The model under review builds one solid part; all positions refer to its coordinate system, in mm. Round coordinates to 2 decimals unless told otherwise and drop trailing zeros. Order: outer loops, then holes, each group sorted by start corner. A loop starts at its lowest first (then second) coordinate and runs counter-clockwise, first axis right, second up.
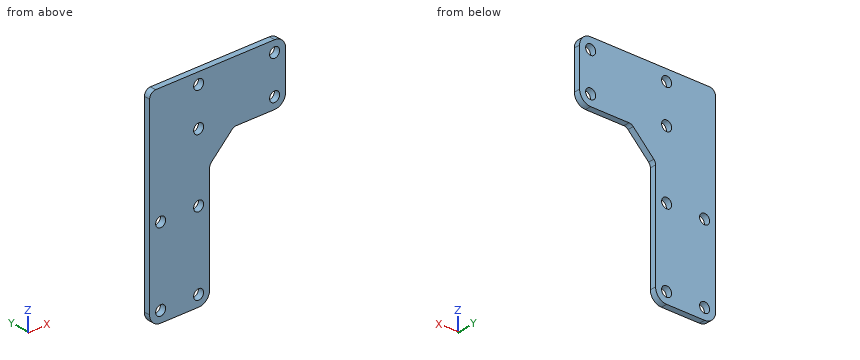
Autodesk Inventor part; units mm, degrees
ref_plane "YZ Plane" through (0, 0, 0) normal (1, 0, 0) x (0, 1, 0)
ref_plane "XZ Plane" through (0, 0, 0) normal (0, 1, 0) x (-1, 0, 0)
ref_plane "XY Plane" through (0, 0, 0) normal (0, 0, 1) x (1, 0, 0)
sketch "Sketch1" plane through (0, 0, 0) normal (0, 1, 0) x (-1, 0, 0)
  circle A0 centre (0, 0) radius 2.63
  line L0 (0, 0) -> (0, -2.63) construction
  line L1 (0, 0) -> (-2.63, 0) construction
  circle A1 centre (0, -20) radius 2.63
  circle A2 centre (-20, 0) radius 2.63 construction
  circle A3 centre (-20, -20) radius 2.63 construction
  circle A4 centre (-40, 0) radius 2.63
  circle A5 centre (-40, -20) radius 2.63
  circle A6 centre (0, -55) radius 2.63
  circle A7 centre (20, -55) radius 2.63
  circle A8 centre (20, -95) radius 2.63
  circle A9 centre (0, -95) radius 2.63
  circle A10 centre (0, 0) radius 5.805 construction
  circle A11 centre (20, -55) radius 5.805 construction
  circle A12 centre (0, -55) radius 5.805 construction
  circle A13 centre (20, -95) radius 5.805 construction
  circle A14 centre (0, -95) radius 5.805 construction
  circle A15 centre (-40, -20) radius 5.805 construction
  circle A16 centre (-40, 0) radius 5.805 construction
  line L2 (25.805, -95) -> (25.805, 2.63)
  line L3 (22.63, 5.805) -> (-40, 5.805)
  line L4 (-45.805, 0) -> (-45.805, -20)
  line L5 (-19.8201, -25.805) -> (-40, -25.805)
  circle A17 centre (-20, -20) radius 5.805 construction
  line L6 (-5.805, -39.8201) -> (-5.805, -95)
  line L7 (20, -100.805) -> (0, -100.805)
  arc A18 (20, -100.805) -> (25.805, -95) centre (20, -95) ccw
  arc A19 (-5.805, -95) -> (0, -100.805) centre (0, -95) ccw
  arc A20 (-45.805, -20) -> (-40, -25.805) centre (-40, -20) ccw
  arc A21 (-40, 5.805) -> (-45.805, 0) centre (-40, 0) ccw
  line L8 (-6.7349, -37.5751) -> (-17.5751, -26.7349)
  arc A22 (-5.805, -39.8201) -> (-6.7349, -37.5751) centre (-8.98, -39.8201) ccw
  arc A23 (-17.5751, -26.7349) -> (-19.8201, -25.805) centre (-19.8201, -28.98) ccw
  arc A24 (25.805, 2.63) -> (22.63, 5.805) centre (22.63, 2.63) ccw
  point P0 (0, -22.63)
  point P1 (-2.63, -20)
  point P2 (-20, -2.63)
  point P3 (-22.63, 0)
  point P4 (-20, -22.63)
  point P5 (-22.63, -20)
  point P6 (-40, -2.63)
  point P7 (-42.63, 0)
  point P8 (-40, -22.63)
  point P9 (-42.63, -20)
  point P10 (-5.805, -25.805)
  point P11 (-5.805, -38.505)
  point P12 (-18.505, -25.805)
  dimension "d0" = 5.26
  dimension "d3" = 20
  dimension "d6" = 20
  dimension "d10" = 20
  dimension "d12" = 75
  dimension "d13" = 40
  dimension "d14" = 3.175
  dimension "d16" = 12.7
  dimension "d17" = 12.7
  dimension "d18" = 3.175
extrude "Extrusion1" add sketch "Sketch1" along normal blind 3.175
properties part number "CNC-013-ZAxisMainMount" material "Aluminum 6061"
(1) To check wall thickness, follow probe 1 along Z at (x, y) = (0, 2.4) (3 decimals); probe 2 along Z at (x, y) = (-20, 0.95) (3 decimals); probe 3 along Z at (x, y) = (40, 2.5) (3 decimals). State the ranges of each line that lie inside material, in increasing order.
Data:
probe 1: z = -100.805 to -97.63, -92.37 to -57.63, -52.37 to -22.63, -17.37 to -2.63, 2.63 to 5.805
probe 2: z = -100.805 to -97.63, -92.37 to -57.63, -52.37 to 5.805
probe 3: z = -25.805 to -22.63, -17.37 to -2.63, 2.63 to 5.805
(2) Consider section A-A (z = -55). Write out the cut boundary in (x, y) (3 decimals), and give its area (3 significant figures).
Data:
outline: (-25.805, 0) - (-22.63, 0) - (-22.63, 3.175) - (-25.805, 3.175) - close; (-17.37, 0) - (-2.63, 0) - (-2.63, 3.175) - (-17.37, 3.175) - close; (2.63, 0) - (5.805, 0) - (5.805, 3.175) - (2.63, 3.175) - close
area: 67.0 mm2
(3) Consider section D-D (x = 13). Write out the cut boundary in (y, z) (3 decimals).
Data:
outline: (0, -31.31) - (3.175, -31.31) - (3.175, 5.805) - (0, 5.805) - close
(4) Insertion check: pin 1 (1 mm diameter, centred on x = 9, y = 1.5, fed in from -Z); pin 2 (1 mm diameter, centred on y = 1.5, z = -59.5, fed in from +X) (3 decimals); pin 3 (1 mm diameter, centred on x = 25.5, y = 2, fed in from -Z) (3 decimals). Each pin has a flat end and moves straight along its axis. Give the tip position at first contact, or say it passes through.
Data:
pin 1: stops at z = -35.81
pin 2: stops at x = 5.805
pin 3: stops at z = -25.805
(5) Consider section B-B (y = 1.85). State how many separate pieces and enclosed holes the cut face has, and give its area (3 significant figures).
Data:
separate pieces: 1
enclosed holes: 8
area: 4,510 mm2
(6) Consider section C-C (x = 38.5). Write out the cut boundary in (y, z) (3 decimals).
Data:
outline: (0, -25.805) - (3.175, -25.805) - (3.175, -22.16) - (0, -22.16) - close; (0, -17.84) - (3.175, -17.84) - (3.175, -2.16) - (0, -2.16) - close; (0, 2.16) - (3.175, 2.16) - (3.175, 5.805) - (0, 5.805) - close
